Check sheet for the modelled part. Datum: model origin and axes. Units: mm. Face numbers are marked on the shaded views. Round coordinates to 2 decimals unless told otherwise and drop trailing zeros. Order: outer loops, then holes, each group sorted by start corner. A loop starts at its lowest first (then second) coordinate and runs counter-clockwise, first axis right, second up.
Q1. Depth check by flat-ended pin: P1, Ø5, axis at y = 22.5, z = -4, coming from the +X side; P2, Ø22, axis at x = 0, z = 0, coming from the -Y side; P3, Ø4, axis at x = -12, y = 19, coming from the +Z side; P4, Ø6, axis at x = -17, y = 3, coming from the -Z side. Enter the tip coordinate at first touch or a pass-through.
Q2. Cross-section at A-A on x = 0. Record the cut outline in (y, z).
Q3. Scan lines: probe 1 along X at (y, z) = (12, 0); probe 2 along Z at (x, y) = (5.5, 11); probe 3 along Z at (x, y) = (-4, 4). Record each from-to range of solid material in increasing order.
Q4. Mould release check, pull along X, two halves, no side actions. Record for the marked faces 1, 2 and 3: +X half, -X half, draft (parallel to the pull), parting line (faces both ways), or undercut.
Q5. Cross-section at C-C on y = 6. Record the cut outline in (x, z).
Q6. Cross-section at B-B on z = 0. Record the cut outline in (x, y).
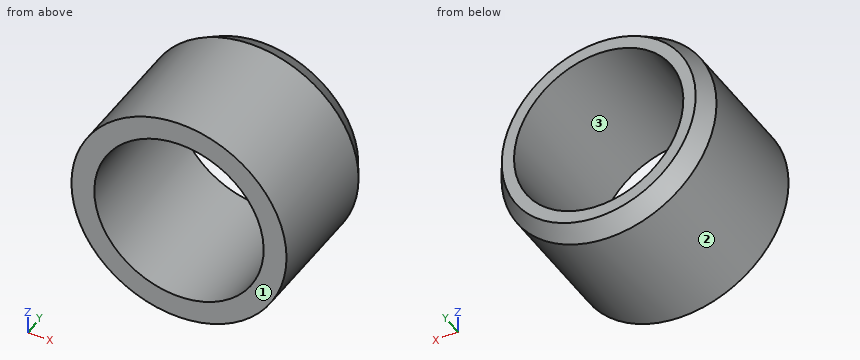
from build123d import *

# Parameters (mm, degrees)
SKETCH1_R           = 23.5
BOSS_EXTRUDE1_DEPTH = 32
SKETCH2_R           = 18.5
CUT_EXTRUDE1_DEPTH  = 32
CHAMFER1_SIZE       = 4
CHAMFER1_SIZE2      = 2.309401077


with BuildPart() as part:
    # Sketch1 → Boss-Extrude1 (new body)
    with BuildSketch(Plane(origin=(0, 0, 0), x_dir=(1, 0, 0), z_dir=(0, 1, 0))):
        with Locations(Location((0, 0, 0), (0, 0, 270))):
            Circle(SKETCH1_R)
    extrude(amount=BOSS_EXTRUDE1_DEPTH)

    # Sketch2 → Cut-Extrude1 (cut)
    with BuildSketch(Plane(origin=(0, 32, 0), x_dir=(1, 0, 0), z_dir=(0, 1, 0))):
        with Locations(Location((0, 0, 0), (0, 0, 270))):
            Circle(SKETCH2_R)
    extrude(amount=-CUT_EXTRUDE1_DEPTH, mode=Mode.SUBTRACT)

    # Chamfer1
    chamfer1_edges = [part.edges().sort_by_distance(p)[0] for p in [
        (0, 32, -23.5),
    ]]
    chamfer1_side = [part.faces().sort_by_distance(p)[0] for p in [
        (0, 16, -23.5),
    ]]
    chamfer(chamfer1_edges, length=CHAMFER1_SIZE, length2=CHAMFER1_SIZE2, reference=chamfer1_side[0])


solid = part.part
Results found:
1. P1: stops at x = 23.45
1. P2: passes through
1. P3: stops at z = 21.27
1. P4: stops at z = -18.87
2. outline: (0, -23.5) - (28, -23.5) - (32, -21.19) - (32, -18.5) - (0, -18.5) - close; (0, 18.5) - (32, 18.5) - (32, 21.19) - (28, 23.5) - (0, 23.5) - close
3. probe 1: x = -23.5 to -18.5, 18.5 to 23.5
3. probe 2: z = -22.85 to -17.66, 17.66 to 22.85
3. probe 3: z = -23.16 to -18.06, 18.06 to 23.16
4. face 1: draft
4. face 2: parting line
4. face 3: undercut
5. outline: circle Ø47 at (0, 0); hole circle Ø37 at (0, 0)
6. outline: (-23.5, 0) - (-18.5, 0) - (-18.5, 32) - (-21.19, 32) - (-23.5, 28) - close; (18.5, 0) - (23.5, 0) - (23.5, 28) - (21.19, 32) - (18.5, 32) - close
